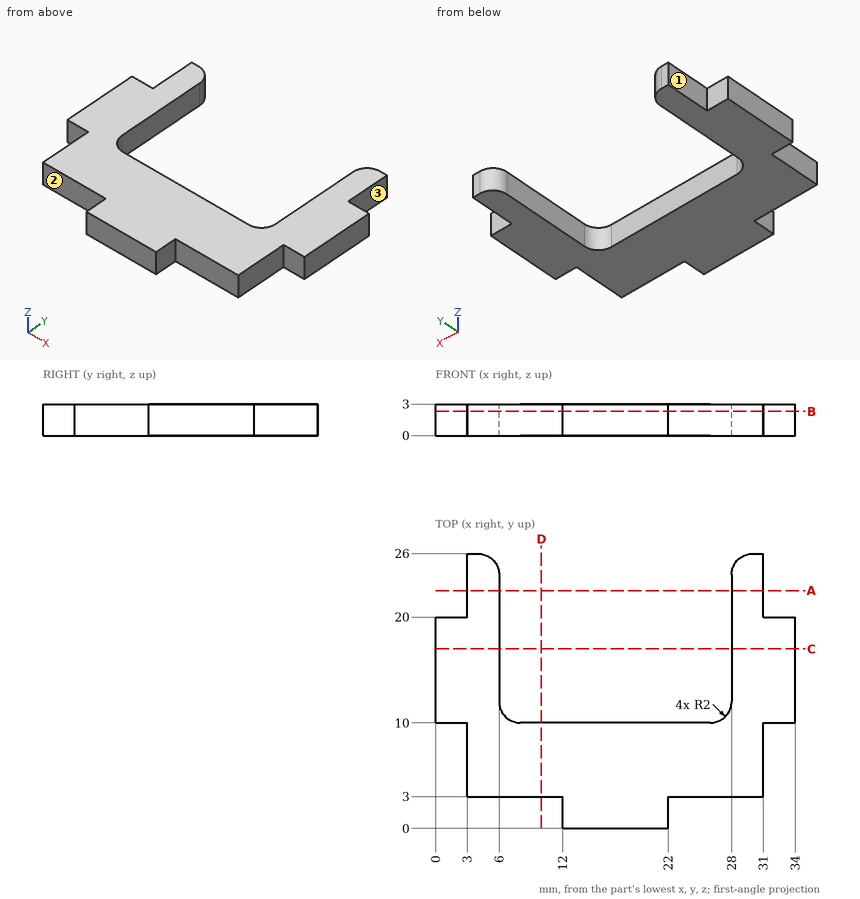
Geometry: see drawing. Coordinates: mm, zero at the bounding-box minimum. A direction names the side the tool comes from. Round coordinates to 2 decimals unless told otherwise and drop trailing zeros. Loops run counter-clockwise (first coordinate to the right, second up) from the corner with the lowest first, then second, coordinate; pieces in that order, holes last. Notation, with made-up numbers: (-40, 41.25) -> (-13, 41.25) arc R26 cw to (-13, 71.25) -> close; hole circle Ø5 at (65.25, -29.75). An arc over 180 degrees is marked (long way). Write each question's results on one line, items separated by ' | '.
1. Section C-C (y = 17). Return loops of the section in (x, z).
Geometry results:
outline: (0, 0) -> (6, 0) -> (6, 3) -> (0, 3) -> close; (28, 0) -> (34, 0) -> (34, 3) -> (28, 3) -> close
2. Ray query, line 1 (X direction, y = 21.5, z = 1.5); line 2 (X direction, y = 15, z = 2.7); line 3 (X direction, y = 5.25, z = 2.6). Return the intervals inside material, ascending. Write a range as from..to.
Geometry results:
line 1: 3..6, 28..31 | line 2: 0..6, 28..34 | line 3: 3..31
3. Set-up query: the marked faces 1, 2 and 3. Return all of +Z, -Z, +X, -X, +Y, -Y with unobstructed straight access to the full face (end or side cutting, diameter ignored); none if empty.
Geometry results:
face 1: +Z, -Z, -X, +Y | face 2: +Z, -Z, -X, -Y | face 3: +Z, -Z, +X, +Y
4. Section B-B (z = 2.3). Return loops of the section in (x, y), and give its area (3 significant figures).
Geometry results:
outline: (0, 10) -> (3, 10) -> (3, 3) -> (12, 3) -> (12, 0) -> (22, 0) -> (22, 3) -> (31, 3) -> (31, 10) -> (34, 10) -> (34, 20) -> (31, 20) -> (31, 26) -> (30, 26) arc R2 ccw to (28, 24) -> (28, 12) arc R2 cw to (26, 10) -> (8, 10) arc R2 cw to (6, 12) -> (6, 24) arc R2 ccw to (4, 26) -> (3, 26) -> (3, 20) -> (0, 20) -> close | area: 382 mm2
5. Section D-D (x = 10). Return loops of the section in (y, z), and give its area (3 significant figures).
Geometry results:
outline: (3, 0) -> (10, 0) -> (10, 3) -> (3, 3) -> close | area: 21.0 mm2
6. First-contact query: P1, Ø0.9, axis at x = 1.5, z = 2, coming from the -Y side; P2, Ø0.9, axis at y = 1.5, z = 2, coming from the -X side; P3, Ø12, axis at x = 16, y = 23.5, coming from the +Z side; P4, Ø1.5, axis at x = 1, z = 1.5, coming from the +Y side. Flat tips, straight axial feed; report the tip coordinate or a pass-through.
Geometry results:
P1: y = 10 | P2: x = 12 | P3: through | P4: y = 20
7. Section A-A (y = 22.5). Return loops of the section in (x, z), and give its area (3 significant figures).
Geometry results:
outline: (3, 0) -> (6, 0) -> (6, 3) -> (3, 3) -> close; (28, 0) -> (31, 0) -> (31, 3) -> (28, 3) -> close | area: 18.0 mm2
